Autodesk Inventor part; units mm, degrees
ref_plane "YZ Plane" through (0, 0, 0) normal (1, 0, 0) x (0, 1, 0)
ref_plane "XZ Plane" through (0, 0, 0) normal (0, 1, 0) x (-1, 0, 0)
ref_plane "XY Plane" through (0, 0, 0) normal (0, 0, 1) x (1, 0, 0)
sketch "Sketch1" plane through (0, 0, 0) normal (0, 0, 1) x (1, 0, 0)
  line L0 (10, -10) -> (-10, -10)
  line L1 (-10, -10) -> (-10, 10)
  line L2 (-10, 10) -> (10, 10)
  line L3 (10, 10) -> (10, -10)
  line L4 (10, -10) -> (-10, 10) construction
  line L5 (-10, -10) -> (10, 10) construction
  line L6 (10, -10) -> (6, -10)
  line L7 (6, 10) -> (10, 10)
  line L8 (10, 10) -> (10, -10)
  line L9 (0, 10) -> (0, -10)
  line L10 (0, -10) -> (0, 10)
  point P0 (0, 0)
  dimension "d0" = 20
  dimension "d1" = 20
extrude "Extrusion1" add sketch "Sketch1" along normal blind 5 contours L0 L9 L2 L3
ref_plane "Work Plane1" through (0, 0, 2.5) normal (0, 0, 1) x (1, 0, 0)
sketch "Sketch2" plane through (0, 0, 2.5) normal (0, 0, 1) x (1, 0, 0)
  line L0 (0, 10) -> (0, -10)
  line L1 (0, 2.8868) -> (2.5, 1.4434)
  line L2 (2.5, 1.4434) -> (2.5, -1.4434)
  line L3 (2.5, -1.4434) -> (0, -2.8868)
  line L4 (0, -2.8868) -> (-2.5, -1.4434)
  line L5 (-2.5, -1.4434) -> (-2.5, 1.4434)
  line L6 (-2.5, 1.4434) -> (0, 2.8868)
  point P0 (0, 0)
  point P1 (0, 0)
  dimension "d12" = 5
extrude "Extrusion2" cut sketch "Sketch2" along normal mid plane 1.8
sketch "Sketch3" plane through (0, 0, 5) normal (0, 0, 1) x (1, 0, 0)
  circle A0 centre (0, 0) radius 1.75
  dimension "d15" = 3.5
extrude "Extrusion3" cut sketch "Sketch3" against normal blind 8
sketch "Sketch4" plane through (10, -10, 0) normal (1, 0, 0) x (0, 0, -1)
  circle A0 centre (-2.5, 17.5) radius 1.3
  circle A1 centre (-2.5, 2.5) radius 1.3
  line L0 (0, 20) -> (-5, 20)
  line L1 (0, 0) -> (-5, 0)
  line L2 (0, 0) -> (0, 20)
  point P0 (0, 10)
  dimension "d18" = 2.5
  dimension "d19" = 2.5
  dimension "d20" = 2.5
  dimension "d21" = 2.5
  dimension "d22" = 2.6
  dimension "d23" = 2.6
extrude "Extrusion4" cut sketch "Sketch4" against normal blind 25
sketch "Sketch5" plane through (10, -10, 0) normal (1, 0, 0) x (0, 0, -1)
  circle A0 centre (-2.5, 17.5) radius 1.3
  circle A1 centre (-2.5, 17.5) radius 2
  circle A2 centre (-2.5, 2.5) radius 1.3
  circle A3 centre (-2.5, 2.5) radius 2
  point P0 (0, 10)
  dimension "d26" = 4
  dimension "d27" = 4
extrude "Extrusion5" cut sketch "Sketch5" against normal blind 4 contours A0 | A1 | A2 | A3
sketch "Sketch6" plane through (0, 0, 5) normal (0, 0, 1) x (1, 0, 0)
  point P0 (0, 0)
sketch "Sketch7" plane through (0, 0, 5) normal (0, 0, 1) x (1, 0, 0)
  line L0 (10, -10) -> (10, 10)
  line L1 (10, 10) -> (5, 10)
  line L2 (5, 10) -> (5, 5)
  line L3 (5, 5) -> (10, 5)
  line L4 (10, 5) -> (10, 10)
  line L5 (0, -10) -> (10, -10)
  line L6 (10, -10) -> (5, -10)
  line L7 (5, -10) -> (5, -5)
  line L8 (5, -5) -> (10, -5)
  line L9 (10, -5) -> (10, -10)
  point P0 (0, 0)
  dimension "d30" = 5
  dimension "d31" = 5
  dimension "d32" = 5
  dimension "d33" = 5
extrude "Extrusion6" cut sketch "Sketch7" against normal blind 10
sketch "Sketch8" plane through (10, -5, 0) normal (1, 0, 0) x (0, 0, -1)
  line L0 (0, 0) -> (5, 0)
  line L1 (5, 0) -> (5, 10)
  line L2 (5, 10) -> (0, 10)
  line L3 (0, 10) -> (0, 0)
  line L4 (-5, 0) -> (-5, 10)
  line L5 (-5, 10) -> (-10, 10)
  line L6 (-10, 10) -> (-10, 0)
  line L7 (-10, 0) -> (-5, 0)
  line L8 (-5, 0) -> (-5, 10)
  circle A0 centre (-7.5, 5) radius 1.375
  circle A1 centre (2.5, 5) radius 1.375
  point P0 (0, 5)
  point P1 (-7.5, 0)
  dimension "d36" = 5
  dimension "d37" = 5
  dimension "d38" = 5
  dimension "d39" = 2.75
  dimension "d40" = 2.75
  dimension "d41" = 5
  dimension "d42" = 5
  dimension "d43" = 5
  dimension "d44" = 5
  dimension "d45" = 2.5
  dimension "d46" = 2.5
extrude "Extrusion7" add sketch "Sketch8" against normal blind 5
sketch "Sketch9" plane through (5, -5, 0) normal (-1, 0, 0) x (0, 0, 1)
  circle A0 centre (7.5, 5) radius 1.375
  circle A1 centre (7.5, 5) radius 2
  circle A2 centre (-2.5, 5) radius 1.375
  circle A3 centre (-2.5, 5) radius 2
  point P0 (0, 5)
  dimension "d49" = 4
  dimension "d50" = 4
extrude "Extrusion8" cut sketch "Sketch9" against normal blind 2 contours A0 | A1 | A2 | A3
equation "\"d18\" = d19"
equation "\"d20\" = d19"
equation "\"d21\" = d19"
equation "\"d23\" = d22"
equation "\"d27\" = d26"
equation "\"d42\" = d41"
equation "\"d50\" = d49"
properties part number "POMSliderMotor"
Geometry: final body of the model. Coordinates: model frame, mm. A direction names the side the tool comes from. Coordinates: 2 decimals unless noted, no trailing zeros. Order: outer loops, then holes, each group sorted by start corner. A loop starts at its lowest first (then second) coordinate and runs counter-clockwise, first axis right, second up.
(1) First-contact query: pin 1 (4 mm diameter, centred on x = 2, y = 3.5, fed in from +Z); pin 2 (4 mm diameter, centred on y = 0, z = -1.5, fed in from -X); pin 3 (2 mm diameter, centred on y = -7.5, z = 2.5, fed in from +X); pin 4 (1.5 mm diameter, centred on x = 7, z = 4, fed in from +Y). Flat tips, straight axial feed; report the tip coordinate or a pass-through.
(2) Section query A-A (z = 2.5). Return the cut outline in (x, y), plus the area to 3 significant figures.
(3) Section query C-C (y = 0). Return the cut outline in (x, z) (3 decimals), plus the area to 3 significant figures.
(4) Draft query along Z for faces 1 (the face through (2, 0, 3.4)), 2 (the face through (5, 2.3, -2.5)), 3 (the face through (8, 0, 10)). Return one class per face: pulls with the +Z half, pulls with the -Z half, needs draft (parallel to the pull), parting line crosses it, or undercut.
(5) Section query B-B (x = 1.25). Return the cut outline in (y, z), plus the area to 3 significant figures.
(6) Material intervals for probe 1 along Y at (x, z) = (4, 2.5); probe 2 along Y at (x, z) = (5.95, 7.5); probe 3 along Y at (x, z) = (1.7, 2.5), sorted ascending.
(7) Section query D-D (z = 7.5). Return the cut outline in (x, y) (3 decimals), plus the area to 4 significant figures.
(8) Access query for faces 4 (the face through (2, 0, 5)), 5 (the face through (2, 10, 2)), 6 (the face through (7, -5, 3)), 7 (the face through (1.267, -2.155, 2.487)). Directions: +Z, -Z, +X, -X, +Y, -Y. A direction counts if a zero-diameter tool reaches every point of the face in a straight line with its end or side. Return the directions, or none.
Solution:
1. pin 1: stops at z = 5
1. pin 2: stops at x = 1.15
1. pin 3: passes through
1. pin 4: stops at y = 5
2. outline: (0, -10) - (5, -10) - (5, -8.8) - (0, -8.8) - close; (0, -6.2) - (5, -6.2) - (5, -5) - (10, -5) - (10, 5) - (5, 5) - (5, 6.2) - (0, 6.2) - (0, 2.89) - (2.5, 1.44) - (2.5, -1.44) - (0, -2.89) - close; (0, 8.8) - (5, 8.8) - (5, 10) - (0, 10) - close
2. area: 113 mm2
3. outline: (1.75, 0) - (5, 0) - (5, -0.5) - (7, -0.5) - (7, -1.125) - (10, -1.125) - (10, 6.125) - (7, 6.125) - (7, 5.5) - (5, 5.5) - (5, 5) - (1.75, 5) - (1.75, 3.4) - (2.5, 3.4) - (2.5, 1.6) - (1.75, 1.6) - close; (5, -5) - (10, -5) - (10, -3.875) - (7, -3.875) - (7, -4.5) - (5, -4.5) - close; (5, 9.5) - (7, 9.5) - (7, 8.875) - (10, 8.875) - (10, 10) - (5, 10) - close
3. area: 57.4 mm2
4. face 1: undercut
4. face 2: needs draft
4. face 3: pulls with the +Z half
5. outline: (-10, 0) - (-1.22, 0) - (-1.22, 1.6) - (-2.17, 1.6) - (-2.17, 3.4) - (-1.22, 3.4) - (-1.22, 5) - (-10, 5) - close; (1.22, 0) - (10, 0) - (10, 5) - (1.22, 5) - (1.22, 3.4) - (2.17, 3.4) - (2.17, 1.6) - (1.22, 1.6) - close; hole circle Ø2.6 at (-7.5, 2.5); hole circle Ø2.6 at (7.5, 2.5)
5. area: 73.7 mm2
6. probe 1: y = -10 to -8.8, -6.2 to 6.2, 8.8 to 10
6. probe 2: y = -5 to -2, 2 to 5
6. probe 3: y = -10 to -8.8, -6.2 to -1.91, 1.91 to 6.2, 8.8 to 10
7. outline: (5, -5) - (10, -5) - (10, -1.375) - (7, -1.375) - (7, -2) - (5, -2) - close; (5, 2) - (7, 2) - (7, 1.375) - (10, 1.375) - (10, 5) - (5, 5) - close
7. area: 33.75 mm2
8. face 4: +Z, -X, +Y, -Y
8. face 5: +Z, -Z, +X, -X, +Y
8. face 6: +Z, -Z, +X, -Y
8. face 7: -X
